Geometry check sheet. Reference: the model listing, model coordinates, mm. Face numbers are marked on the shaded views. A direction names the side the tool comes from. Coordinates: 2 decimals unless noted, no trailing zeros. Write each loop counter-clockwise with the first axis right and the second up, starting at its lowest first coordinate (ties: lowest second). Pieces come first, ordered by that corner, then holes. Notation, with made-up numbers: (-32, -12) -> (-3, -12) arc R15 cw to (-3, 6) -> close; hole circle Ø11 at (-7.5, 14). An arc over 180 degrees is marked (long way). Put each result on its own line as item: value. Start each with the question number.
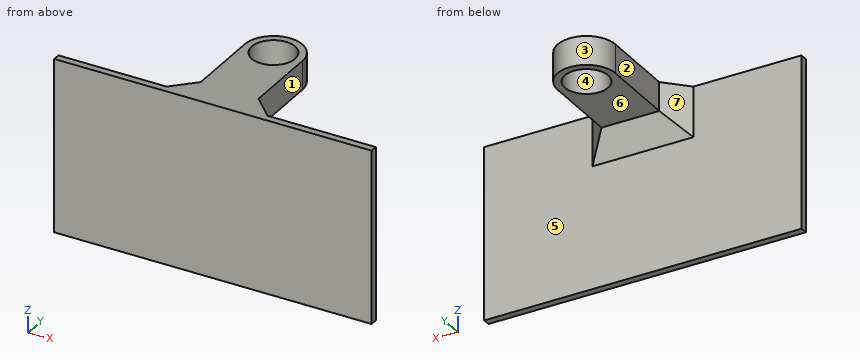
from build123d import *

# Parameters (mm, degrees)
ESBO_O1_W                = 220
ESBO_O1_H                = 120
RESSALTO_EXTRUS_O1_DEPTH = 5
ESBO_O2_R                = 15
RESSALTO_EXTRUS_O2_DEPTH = 20
CHANFRO1_SIZE            = 15


with BuildPart() as part:
    # Esboço1 → Ressalto-extrusão1 (new body)
    with BuildSketch(Plane(origin=(0, 0, 0), x_dir=(1, 0, 0), z_dir=(0, 1, 0))):
        Rectangle(ESBO_O1_W, ESBO_O1_H)
    extrude(amount=RESSALTO_EXTRUS_O1_DEPTH)

    # Esboço2 → Ressalto-extrusão2 (add)
    with BuildSketch(Plane.XY.offset(60)):
        with BuildLine():
            Line((20, 72.5), (20, 5))
            Line((20, 5), (-20, 5))
            Line((-20, 5), (-20, 72.5))
            ThreePointArc((-20, 72.5), (0, 92.5), (20, 72.5))
        make_face()
        with Locations((0, 72.5)):
            Circle(ESBO_O2_R, mode=Mode.SUBTRACT)
    extrude(amount=-RESSALTO_EXTRUS_O2_DEPTH)

    # Chanfro1
    chanfro1_edges = [part.edges().sort_by_distance(p)[0] for p in [
        (0, 5, 40),
        (20, 5, 50),
        (-20, 5, 50),
    ]]
    chamfer(chanfro1_edges, length=CHANFRO1_SIZE)


solid = part.part
Item 1: Section check B-B, the plane z = 45. Enter the section's corners in (x, y), and give its area (3 significant figures).
Item 2: Section check D-D, the plane z = -47.5. Enter the section's corners in (x, y), and give its area (3 significant figures).
Item 3: Go/stop test with flat-tipped pins: P1, Ø10, axis at y = 54.5, z = 45.5, coming from the -X side; P2, Ø8, axis at x = 4.5, y = 58, coming from the -Z side; P3, Ø6, axis at y = 35, z = 50, coming from the +X side. Record where each tip stops, or that it passes through.
Item 4: Scan lines: line 1 along Y through (x, z) = (0, 49.25); line 2 along Y through (x, z) = (-14, 0); line 3 along Z through (x, y) = (-15.5, 67). Record each from-to range of solid material in increasing order. Write a range as [from, to].
Item 5: Mould release check, pull along X, two halves, no side actions. Record for the marked faces 1, 2, 3 and 4: released by +X, released by -X, zero draft, split by the parting line, or undercut.
Item 6: Access from +Z, -Z, +X, -X, +Y, -Y to the whole of each face (thin tool, end or side, straight path). Record for the marked faces 5, 6 and 7.
Item 7: Section check C-C, the plane y = 68. Enter the section's corners in (x, z), and give its area (3 significant figures).
Item 8: Section check A-A, the plane x = 0. Enter the section's corners in (y, z).
From the geometry:
1. outline: (-110, 0) -> (110, 0) -> (110, 5) -> (35, 5) -> (20, 20) -> (20, 72.5) arc R20 ccw to (-20, 72.5) -> (-20, 20) -> (-35, 5) -> (-110, 5) -> close; hole circle Ø30 at (0, 72.5)
1. area: 3,950 mm²
2. outline: (-110, 0) -> (110, 0) -> (110, 5) -> (-110, 5) -> close
2. area: 1,100 mm²
3. P1: x = -20
3. P2: z = 40
3. P3: x = 20
4. line 1: [0, 57.5], [87.5, 92.5]
4. line 2: [0, 5]
4. line 3: [40, 60]
5. face 1: released by +X
5. face 2: released by -X
5. face 3: split by the parting line
5. face 4: undercut
6. face 5: -Z, +Y
6. face 6: -Z, +X, -X, +Y
6. face 7: +Z, -Z, -X, +Y
7. outline: (-20, 40) -> (-14.31, 40) -> (-14.31, 60) -> (-20, 60) -> close; (14.31, 40) -> (20, 40) -> (20, 60) -> (14.31, 60) -> close
7. area: 228 mm²
8. outline: (0, -60) -> (5, -60) -> (5, 25) -> (20, 40) -> (57.5, 40) -> (57.5, 60) -> (0, 60) -> close; (87.5, 40) -> (92.5, 40) -> (92.5, 60) -> (87.5, 60) -> close
